Input: dimensioned drawing with shaded views. Units: mm. Origin: part minimum x, y, z. A direction names the side the tool comes from. Give positions to 0.01 mm unless a question says otherwise; leave off trailing zeros. Order: outer loops, then holes, each group sorted by start corner. A loop starts at its lowest first (then second) coordinate and runs counter-clockwise, first axis right, second up. Notation, with made-up numbers: (8.25, -11.75) -> (31.25, -11.75) arc R35 ccw to (31.25, 25.25) -> close; hole circle Ø10 at (-3, 85.25). An arc over 180 degrees is marked (long way). One line per question, with ' | ' between items. Start each with the question number.
(1) Ray query, L1, parallel to Z at x = 9, y = 1.75; L2, parallel to Z at x = 6.5, y = 7.75; L3, parallel to X at y = 7.5, z = 4.6. Return the intervals inside material, ascending.
(2) First-contact query: pin 1 Ø2 at (x, z) = (15.5, 1.5) entering from -Y. Flat tip, straight axial feed; report the tip coordinate or a pass-through.
(3) Mould query, pull axis X, two halves, no side actions, for the marked faces 3 and 4. Classes: +X half, -X half, draft (parallel to the pull), parting line (faces both ways), or undercut.
(4) Section A-A (x = 9). Return loops of the section in (y, z), then the cut area to 3 significant figures.
(5) Set-up query: the marked faces 1 and 2. Return all of +Z, -Z, +X, -X, +Y, -Y with unobstructed straight access to the full face (end or side cutting, diameter ignored); none if empty.
(6) Section D-D (y = 12). Return loops of the section in (x, z).
(7) Section C-C (z = 3.6). Return loops of the section in (x, y).
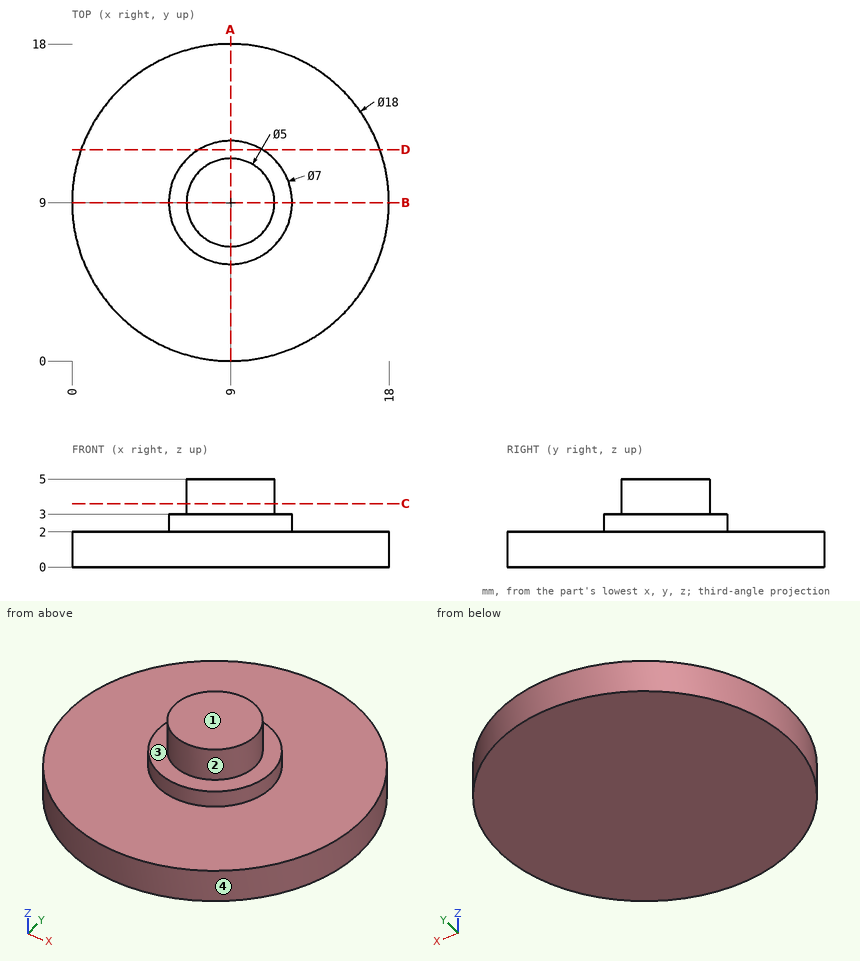
Response:
1) L1: z = 0 to 2 | L2: z = 0 to 3 | L3: x = 7 to 11
2) pin 1: stops at y = 1.88
3) face 3: draft | face 4: parting line
4) outline: (0, 0) -> (18, 0) -> (18, 2) -> (12.5, 2) -> (12.5, 3) -> (11.5, 3) -> (11.5, 5) -> (6.5, 5) -> (6.5, 3) -> (5.5, 3) -> (5.5, 2) -> (0, 2) -> close | area: 53.0 mm^2
5) face 1: +Z, +X, -X, +Y, -Y | face 2: +Z
6) outline: (0.51, 0) -> (17.49, 0) -> (17.49, 2) -> (10.8, 2) -> (10.8, 3) -> (7.2, 3) -> (7.2, 2) -> (0.51, 2) -> close
7) outline: circle Ø5 at (9, 9)
